Verification items for this drawing (mm, ordinates from the low corner). A direction names the side the tool comes from. Give positions to 0.01 mm unless a question says otherwise; leave off trailing zeros. Write each loop counter-clockwise with the first axis right and the second up, starting at its lowest first coordinate (ties: lowest second). Pieces come first, ordered by that corner, then holes. Notation, with made-up numbers: (-8.5, 31.25) -> (44.5, 31.25) arc R16 cw to (44.5, 47.25) -> close; hole circle Ø11 at (-36.5, 21). An arc over 180 degrees is marked (long way). Use one line per item in the form item = value. Start each with the question number.
(1) Section check D-D, the plane z = 17. Record the cut outline in (x, y) (1 decimal), plus the area to 3 significant figures.
(2) Set-up check for the marked faces 1 and 2: record each of +Z, -Z, +X, -X, +Y, -Y from which the full face is reachable in a straight line by a thin tool's end or side.
(3) Section check B-B, the plane y = 12.7. Record the cut outline in (x, z) (1 decimal).
(4) Scan line: L1, parallel to Z at x = 12.7, y = 0.75. Record every from-to range of solid material in increasing order.
(5) Section check A-A, the plane z = 12.7. Record the cut outline in (x, y) (1 decimal).
(6) Depth check by flat-ended pin: pin 1 Ø6 at (x, y) = (21.5, 6) entering from +Z; pin 2 Ø5.5 at (x, z) = (12.7, 12.7) entering from +Y (3 decimals); pin 3 Ø10 at (x, y) = (9.5, 10.5) entering from +Z; pin 4 Ø11 at (y, z) = (19, 11) entering from +X (3 decimals). Enter the tip coordinate at first touch or a pass-through.
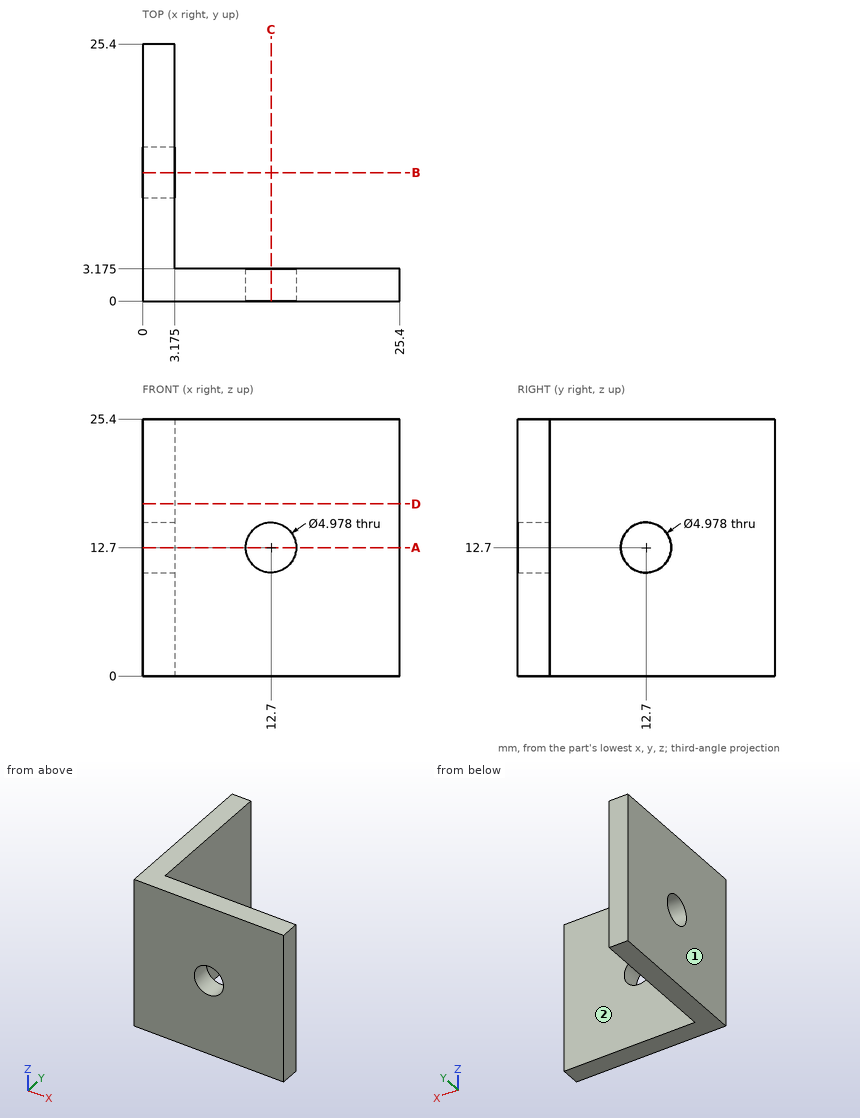
Completed:
q1.outline = (0, 0) -> (25.4, 0) -> (25.4, 3.2) -> (3.2, 3.2) -> (3.2, 25.4) -> (0, 25.4) -> close
q1.area = 151 mm²
q2.face_1 = +Z, -Z, -X, +Y, -Y
q2.face_2 = +Z, -Z, +X, +Y
q3.outline = (0, 0) -> (3.2, 0) -> (3.2, 10.2) -> (0, 10.2) -> close; (0, 15.2) -> (3.2, 15.2) -> (3.2, 25.4) -> (0, 25.4) -> close
q4.L1 = 0 to 10.21, 15.19 to 25.4
q5.outline = (0, 0) -> (10.2, 0) -> (10.2, 3.2) -> (3.2, 3.2) -> (3.2, 10.2) -> (0, 10.2) -> close; (0, 15.2) -> (3.2, 15.2) -> (3.2, 25.4) -> (0, 25.4) -> close; (15.2, 0) -> (25.4, 0) -> (25.4, 3.2) -> (15.2, 3.2) -> close
q6.pin_1 = 25.4
q6.pin_2 = 3.175
q6.pin_3 = through
q6.pin_4 = 3.175
